```python
from build123d import *

# Parameters (mm, degrees)
BOSS_EXTRUDE1_DEPTH = 3.175
CUT_EXTRUDE2_DEPTH  = 3.175
FILLET2_R           = 6.35
SKETCH5_W           = 50.8
SKETCH5_H           = 3.175
BOSS_EXTRUDE2_DEPTH = 4.7625
SKETCH6_W           = 2.38125
SKETCH6_H           = 50.8
CUT_EXTRUDE3_DEPTH  = 223.661605403


with BuildPart() as part:
    # Sketch2 → Boss-Extrude1 (new body)
    with BuildSketch(Plane(origin=(0, 0, 0), x_dir=(1, 0, 0), z_dir=(0, 1, 0))):
        Polygon((0, 0), (-90.9828, 0), (-12.7, 203.2), (0, 203.2), align=None)
    extrude(amount=BOSS_EXTRUDE1_DEPTH)

    # Sketch3 → Cut-Extrude2 (cut)
    with BuildSketch(Plane(origin=(0, 3.175, 0), x_dir=(1, 0, 0), z_dir=(0, 1, 0))):
        Polygon((-19.05, 19.05), (-19.05, 133.726180748), (-63.228998633, 19.05), align=None)
    extrude(amount=-CUT_EXTRUDE2_DEPTH, mode=Mode.SUBTRACT)

    # Fillet2
    fillet2_edges = [part.edges().sort_by_distance(p)[0] for p in [
        (-19.05, 1.5875, -19.05),
        (-63.228998633, 1.5875, -19.05),
        (-19.05, 1.5875, -133.726180748),
    ]]
    fillet(fillet2_edges, radius=FILLET2_R)

    # Sketch5 → Boss-Extrude2 (add)
    with BuildSketch(Plane.XY):
        with Locations((-50.673, 1.5875)):
            Rectangle(SKETCH5_W, SKETCH5_H)
    extrude(amount=BOSS_EXTRUDE2_DEPTH)

    # Sketch6 → Cut-Extrude3 (cut, through all)
    with BuildSketch(Plane(origin=(0, 3.175, 0), x_dir=(1, 0, 0), z_dir=(0, 1, 0))):
        with Locations((-1.190625, 177.8)):
            Rectangle(SKETCH6_W, SKETCH6_H)
    extrude(amount=-CUT_EXTRUDE3_DEPTH, mode=Mode.SUBTRACT)


solid = part.part
```
Part model, mm, in its own coordinate system. A direction names the side the tool comes from. Round coordinates to 2 decimals unless told otherwise and drop trailing zeros. Loops run counter-clockwise (first coordinate to the right, second up) from the corner with the lowest first, then second, coordinate; pieces in that order, holes last. Notation, with made-up numbers: (32.25, 9.25) -> (53.25, 9.25) arc R21 ccw to (53.25, 45.25) -> close; hole circle Ø6 at (-20.5, -16.5). An arc over 180 degrees is marked (long way). Use one line per item in the form item = value. Start each with the question number.
Item 1: Band-saw the part on D-D (x = -9.5). List the corners of the cut face in (y, z) (3 decimals), plus the area to 3 significant figures.
Item 2: Drop flat-ended pins along their axis: pin 1 Ø1 at (x, y) = (-83, 2) entering from +Z; pin 2 Ø12 at (x, z) = (-44.5, -73) entering from -Y; pin 3 Ø1 at (y, z) = (1, 1.5) entering from +X. Give the stop position or say it passes through.
Item 3: Two-plate mould, pull along Z, no slides. Class faces 1 (the flat face through (-45.414, 1.61, -65.292)), 2 (the flat face through (-52.39, 1.57, -100.18)), 3 (the flat face through (-45, 3.175, -78)): released by +Z, released by -Z, zero draft, split by the parting line, or undercut.
Item 4: Tool access for faces 4 (the flat face through (-45, 0, -78)), 5 (the cylindrical face through (-24.36, 1.565, -105.844)): list every direction of +Z, -Z, +X, -X, +Y, -Y with a clear straight run to the whole face (end or side of a thin tool).
Item 5: Drill centre lines: line 1 along X through (y, z) = (1.6, -78.5); line 2 along X through (y, z) = (2.7, -33.5); line 3 along X through (y, z) = (0.7, -116). Where is each one in solid material? Low to high.
Item 6: Band-saw the part on B-B (z = -61). List the corners of the cut face in (x, y) (3 decimals).
Item 7: Band-saw the part on C-C (y = 1.65). List the corners of the cut face in (x, z).
Data:
q1.outline = (0, -203.2) -> (3.175, -203.2) -> (3.175, 0) -> (0, 0) -> close
q1.area = 645 mm^2
q2.pin_1 = 0
q2.pin_2 = 0
q2.pin_3 = -25.27
q3.face_1 = undercut
q3.face_2 = released by -Z
q3.face_3 = zero draft
q4.face_4 = +Z, -Z, +X, -X, -Y
q4.face_5 = +Y, -Y
q5.line_1 = -60.74 to -40.33, -19.05 to 0
q5.line_2 = -78.08 to -57.66, -19.05 to 0
q5.line_3 = -46.29 to 0
q6.outline = (-67.483, 0) -> (-47.068, 0) -> (-47.068, 3.175) -> (-67.483, 3.175) -> close; (-19.05, 0) -> (0, 0) -> (0, 3.175) -> (-19.05, 3.175) -> close
q7.outline = (-90.98, 0) -> (-12.7, -203.2) -> (-2.38, -203.2) -> (-2.38, -152.4) -> (0, -152.4) -> (0, 0) -> (-25.27, 0) -> (-25.27, 4.76) -> (-76.07, 4.76) -> (-76.07, 0) -> close; hole (-59.9, -27.68) -> (-31.33, -101.86) arc R6.35 ccw to (-19.05, -99.58) -> (-19.05, -25.4) arc R6.35 ccw to (-25.4, -19.05) -> (-53.98, -19.05) arc R6.35 ccw to start
